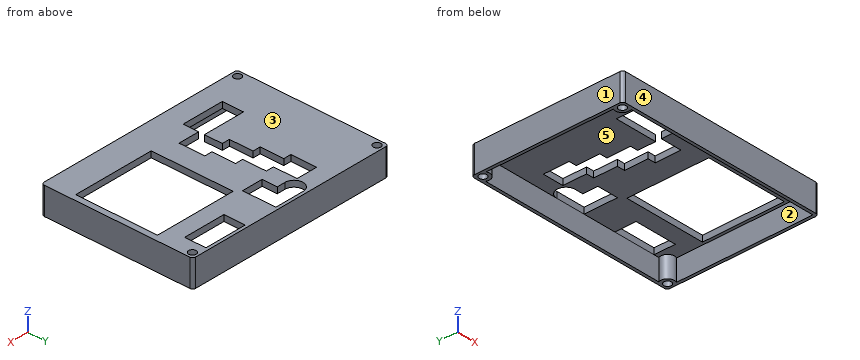
from build123d import *

# Parameters (mm, degrees)
SKETCH2_W           = 70
SKETCH2_H           = 50
SKETCH2_R           = 1.25
SKETCH2_W_2         = 27
SKETCH2_H_2         = 27
SKETCH2_W_3         = 14
SKETCH2_H_3         = 7
BOSS_EXTRUDE1_DEPTH = 2
SKETCH4_W           = 70
SKETCH4_H           = 50
SKETCH4_R           = 1.25
BOSS_EXTRUDE2_DEPTH = 7
FILLET1_R           = 1


with BuildPart() as part:
    # Sketch2 → Boss-Extrude1 (new body)
    with BuildSketch(Plane.XY):
        Rectangle(SKETCH2_W, SKETCH2_H)
        with Locations((-33, 23)):
            Circle(SKETCH2_R, mode=Mode.SUBTRACT)
        with Locations((33, 23)):
            Circle(SKETCH2_R, mode=Mode.SUBTRACT)
        with Locations((-33, -23)):
            Circle(SKETCH2_R, mode=Mode.SUBTRACT)
        with Locations((19.5, -2)):
            Rectangle(SKETCH2_W_2, SKETCH2_H_2, mode=Mode.SUBTRACT)
        Polygon((-22.13, -11), (-8.13, -11), (-8.13, -5.1), (-10.67, -5.1), (-10.67, 2.7), (-13.21, 2.7), (-13.21, 10.5), (-15.75, 10.5), (-15.75, 19), (-8.75, 19), (-8.75, 11.2), (-6.21, 11.2), (-6.21, 3.4), (-3.67, 3.4), (-3.67, -4.4), (-1.13, -4.4), (-1.13, -12.9), (-8.13, -12.9), (-8.13, -18), (-22.13, -18), align=None, mode=Mode.SUBTRACT)
        with BuildLine():
            Line((-2.75, 24), (4.25, 24))
            Line((4.25, 24), (4.25, 13))
            Line((4.25, 13), (-2.75, 13))
            Line((-2.75, 13), (-2.75, 18))
            Line((-2.75, 18), (-5.5, 18))
            ThreePointArc((-5.5, 18), (-8.5, 21), (-5.5, 24))
            Line((-5.5, 24), (-2.75, 24))
        make_face(mode=Mode.SUBTRACT)
        with Locations((22.25, 20.5)):
            Rectangle(SKETCH2_W_3, SKETCH2_H_3, mode=Mode.SUBTRACT)
    extrude(amount=BOSS_EXTRUDE1_DEPTH)

    # Sketch4 → Boss-Extrude2 (add)
    with BuildSketch(Plane(origin=(0, 0, 0), x_dir=(-1, 0, 0), z_dir=(0, 0, -1))):
        Rectangle(SKETCH4_W, SKETCH4_H)
        with Locations((-33, 23)):
            Circle(SKETCH4_R, mode=Mode.SUBTRACT)
        with Locations((33, 23)):
            Circle(SKETCH4_R, mode=Mode.SUBTRACT)
        with Locations((33, -23)):
            Circle(SKETCH4_R, mode=Mode.SUBTRACT)
        with BuildLine():
            Line((-30.984435563, 24), (30.984435563, 24))
            ThreePointArc((30.984435563, 24), (31.409009742, 21.409009742), (34, 20.984435563))
            Line((34, 20.984435563), (34, -20.984435563))
            ThreePointArc((34, -20.984435563), (31.409009742, -21.409009742), (30.984435563, -24))
            Line((30.984435563, -24), (-34, -24))
            Line((-34, -24), (-34, 20.984435563))
            ThreePointArc((-34, 20.984435563), (-31.409009742, 21.409009742), (-30.984435563, 24))
        make_face(mode=Mode.SUBTRACT)
    extrude(amount=BOSS_EXTRUDE2_DEPTH)

    # Fillet1
    fillet1_edges = [part.edges().sort_by_distance(p)[0] for p in [
        (35, -25, -2.5),
        (-35, -25, -2.5),
        (-35, 25, -2.5),
        (35, 25, -2.5),
    ]]
    fillet(fillet1_edges, radius=FILLET1_R)


solid = part.part
The listing builds one solid part. Answer for the finished solid, in the listing's coordinates (mm). Face numbers are marked on the shaded views. A direction names the side the tool comes from. Give positions to 0.01 mm unless a question says otherwise; leave off trailing zeros. Order: outer loops, then holes, each group sorted by start corner. A loop starts at its lowest first (then second) coordinate and runs counter-clockwise, first axis right, second up. Notation, with made-up numbers: (-36.5, 51) -> (-12.5, 51) arc R27 cw to (-12.5, 89) -> close; hole circle Ø4 at (67.5, -37.5). An arc over 180 degrees is marked (long way). Put each result on its own line as item: value.
Item 1: A cutting plane is placed at D-D on z = -4.75. Give the vertices of the cut face in (x, y).
Established:
outline: (-35, -24) arc R1 ccw to (-34, -25) -> (34, -25) arc R1 ccw to (35, -24) -> (35, 24) arc R1 ccw to (34, 25) -> (-34, 25) arc R1 ccw to (-35, 24) -> close; hole circle Ø2.5 at (-33, -23); hole circle Ø2.5 at (-33, 23); hole (-34, -20.98) arc R2.25 cw to (-30.98, -24) -> (34, -24) -> (34, 20.98) arc R2.25 cw to (30.98, 24) -> (-30.98, 24) arc R2.25 cw to (-34, 20.98) -> close; hole circle Ø2.5 at (33, 23)
Item 2: Given P1, Ø2, axis at x = -33, y = -23, coming from the +Z side; P2, Ø24, axis at x = -8, y = 0, coming from the -Z side, each flat-ended and moving along its own axis, determine where each tip first touches the part or whether it passes through.
Established:
P1: passes through
P2: stops at z = 0
Item 3: For the marked faces 1 and 2, determine the directions among +Z, -Z, +X, -X, +Y, -Y from which every point of the face is accessible in a straight line to the end or side of a thin tool.
Established:
face 1: +Z, -Z, -X, +Y, -Y
face 2: -Z
Item 4: Straight lines are drawn through the part: line 1 (X direction, y = 23, z = -3); line 2 (Y direction, x = 22.5, z = 0.75); line 3 (X direction, y = -1, z = 0.5). For each, find the intervals that lie inside material, in ascending order.
Established:
line 1: x = -35 to -34.25, -31.75 to -30.75, 30.75 to 31.75, 34.25 to 35
line 2: y = -25 to -15.5, 11.5 to 17, 24 to 25
line 3: x = -35 to -10.67, -3.67 to 6, 33 to 35
Item 5: For a pull along Y with two mould halves and no side action, classify the marked faces 3, 4 and 5 as released by +Y, released by -Y, zero draft, split by the parting line, or undercut.
Established:
face 3: zero draft
face 4: released by -Y
face 5: undercut
Item 6: A cutting plane is placed at B-B on y = -23. Give the vertices of the cut face in (x, z), plus the area to 3 significant figures.
Established:
outline: (-35, -7) -> (-34.25, -7) -> (-34.25, 2) -> (-35, 2) -> close; (-31.75, -7) -> (-30.75, -7) -> (-30.75, 0) -> (34, 0) -> (34, -7) -> (35, -7) -> (35, 2) -> (-31.75, 2) -> close
area: 154 mm^2
Item 7: A cutting plane is placed at A-A on x = 26.5. Give the vertices of the cut face in (y, z).
Established:
outline: (-25, -7) -> (-24, -7) -> (-24, 0) -> (-15.5, 0) -> (-15.5, 2) -> (-25, 2) -> close; (11.5, 0) -> (17, 0) -> (17, 2) -> (11.5, 2) -> close; (24, -7) -> (25, -7) -> (25, 2) -> (24, 2) -> close
Item 8: A cutting plane is placed at C-C on y = -14.5. Give the vertices of the cut face in (x, z).
Established:
outline: (-35, -7) -> (-34, -7) -> (-34, 0) -> (-22.13, 0) -> (-22.13, 2) -> (-35, 2) -> close; (-8.13, 0) -> (6, 0) -> (6, 2) -> (-8.13, 2) -> close; (33, 0) -> (34, 0) -> (34, -7) -> (35, -7) -> (35, 2) -> (33, 2) -> close
